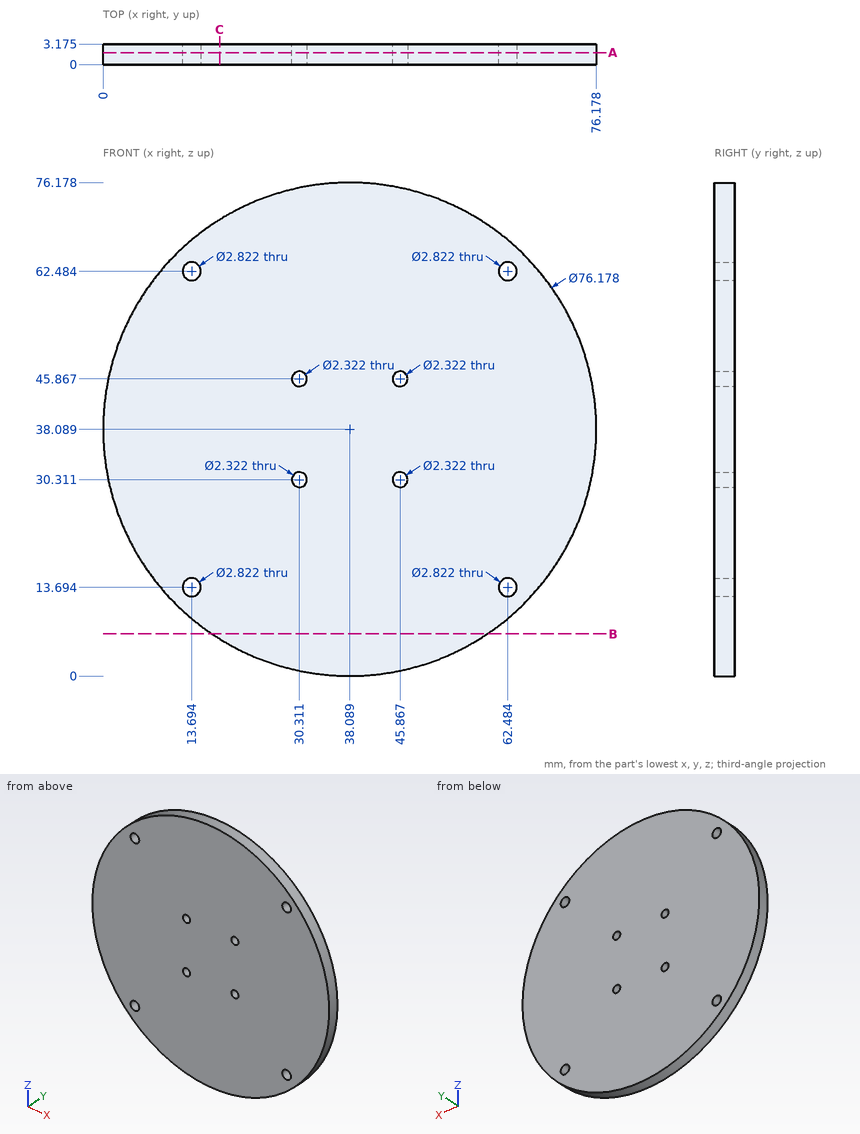
The drawing under review shows one solid part. Ordinate dimensions are in mm from its lowest x, y, z. Coordinates: 2 decimals unless noted, no trailing zeros. Order: outer loops, then holes, each group sorted by start corner. A loop starts at its lowest first (then second) coordinate and runs counter-clockwise, first axis right, second up. Notation, with made-up numbers: (41.5, 50.25) -> (48.5, 50.25) arc R23 cw to (48.5, 89.25) -> close; hole circle Ø10 at (59.5, 32). An arc over 180 degrees is marked (long way). One line per item, written item: value.
1) We need section B-B, the plane z = 6.5. Give the boundary of the cut face in (x, y) (1 decimal).
Output values:
outline: (16.8, 0) -> (59.4, 0) -> (59.4, 3.2) -> (16.8, 3.2) -> close
2) We need section C-C, the plane x = 18. Give the boundary of the cut face in (y, z) (1 decimal).
Output values:
outline: (0, 5.7) -> (3.2, 5.7) -> (3.2, 70.4) -> (0, 70.4) -> close
3) To check wall thickness, follow probe 1 along X at (y, z) = (0.9, 13) (1 decimal); probe 2 along X at (y, z) = (2.6, 10.5); probe 3 along X at (y, z) = (2.6, 7) (1 decimal). State the ranges of each line that lie inside material, in increasing order. Write a range as [from, to].
Output values:
probe 1: x = [9.4, 12.5], [14.9, 61.3], [63.7, 66.7]
probe 2: x = [11.83, 64.35]
probe 3: x = [16.1, 60.1]
4) We need section A-A, the plane y = 1.85. Count the separate pieces of the cut face and the enclosed holes in it, then the cut area to 3 significant figures.
Output values:
separate pieces: 1
enclosed holes: 8
area: 4,520 mm2
5) Clearance check with flat-ended pins moving along their axes: P1, Ø2, axis at x = 53, z = 15, coming from the -Y side; P2, Ø2.5, axis at x = 62.48, z = 62.48, coming from the -Y side; P3, Ø1.5, axis at y = 1.5, z = 15, coming from the -X side. State where each tip first meets the part, or that it passes through.
Output values:
P1: stops at y = 0
P2: passes through
P3: stops at x = 7.24
